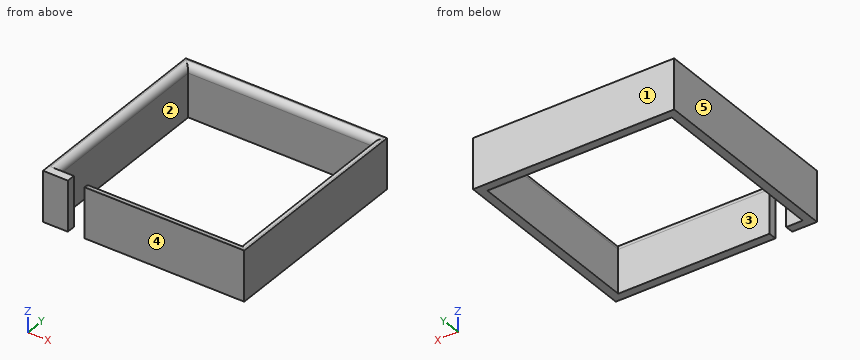
from build123d import *

# Parameters (mm, degrees)
F0_W     = 152.4
F0_H     = 152.4
F0_W_2   = 139.7
F0_H_2   = 139.7
F1_DEPTH = 38.1
F2_W     = 12.7
F2_H     = 38.1
F3_DEPTH = 37.084
F4_R     = 5.08


with BuildPart() as f1:
    # F0 (on Top) → F1 (new body)
    with BuildSketch(Plane.XY):
        with Locations((0, -7.475798)):
            Rectangle(F0_W, F0_H)
        with Locations((0, -7.475798)):
            Rectangle(F0_W_2, F0_H_2, mode=Mode.SUBTRACT)
    extrude(amount=F1_DEPTH)

    # F2 (on face) → F3 (cut)
    with BuildSketch(Plane.XZ.offset(83.675798)):
        with Locations((-51.042333, 19.05)):
            Rectangle(F2_W, F2_H)
    extrude(amount=-F3_DEPTH, mode=Mode.SUBTRACT)

    # F4
    f4_edges = [f1.edges().sort_by_distance(p)[0] for p in [
        (69.85, -7.475798, 38.1),
        (0, 62.374202, 38.1),
        (12.578834, -77.325798, 38.1),
        (-69.85, -7.475798, 38.1),
    ]]
    fillet(f4_edges, radius=F4_R)


solid = f1.part
Could you check a few things on this model? Use its own coordinates, in mm. Face numbers are marked on the shaded views. A direction names the side the tool comes from. Give positions to 0.01 mm unless a question says otherwise; leave off trailing zeros. Write each loop counter-clockwise with the first axis right and the second up, starting at its lowest first coordinate (ties: lowest second). Pieces come first, ordered by that corner, then holes. Notation, with made-up numbers: (-13, 64) -> (5, 64) arc R9 ccw to (5, 68) -> close; hole circle Ø7 at (76.5, 16). An arc over 180 degrees is marked (long way). Answer as CSV lines item,"result". Start each with the question number.
(1) If we section it at B-B, the plane y = -7: Write out the boundary of the cut face in (x, z).
(2) Please list where these lines run through material, in increasing order: line 1 (X direction, y = -10, z = 31); line 2 (Y direction, x = 30.5, z = 27.5); line 3 (Y direction, x = 69, z = 34.5).
(3) If we section it at C-C, the plane z = 16: Write out the boundary of the cut face in (x, y), and give its area (3 significant figures).
(4) Which directions (+Z, -Z, +X, -X, +Y, -Y) give clear straight access to the entire face, cutting with the end or side of a thin tool? Please do the marked faces 1 and 2.
(5) If we section it at A-A, the plane x = -32.5: Write out the boundary of the cut face in (y, z).
(6) If we mould it in two halves opening along Y, with no side actions, what happens to the marked faces 3, 4 and 5? For each: +Y half, -Y half, draft (parallel to the pull), parting line (faces both ways), or undercut.
Answer list:
1,outline,"(-76.2, 0) -> (-69.85, 0) -> (-69.85, 33.02) arc R5.08 ccw to (-74.93, 38.1) -> (-76.2, 38.1) -> close; (69.85, 0) -> (76.2, 0) -> (76.2, 38.1) -> (74.93, 38.1) arc R5.08 ccw to (69.85, 33.02) -> close"
2,line 1,"-76.2 to -69.85, 69.85 to 76.2"
2,line 2,"-83.68 to -77.33, 62.37 to 68.72"
2,line 3,"-83.68 to -77.55, 62.59 to 68.72"
3,outline,"(-76.2, -83.68) -> (-57.39, -83.68) -> (-57.39, -77.33) -> (-69.85, -77.33) -> (-69.85, 62.37) -> (69.85, 62.37) -> (69.85, -77.33) -> (-44.69, -77.33) -> (-44.69, -83.68) -> (76.2, -83.68) -> (76.2, 68.72) -> (-76.2, 68.72) -> close"
3,area,"3,630 mm^2"
4,face 1,"+Z, -Z, +X, -X, +Y"
4,face 2,"+Z, -Z"
5,outline,"(-83.68, 0) -> (-77.33, 0) -> (-77.33, 33.02) arc R5.08 ccw to (-82.41, 38.1) -> (-83.68, 38.1) -> close; (62.37, 0) -> (68.72, 0) -> (68.72, 38.1) -> (67.45, 38.1) arc R5.08 ccw to (62.37, 33.02) -> close"
6,face 3,"undercut"
6,face 4,"-Y half"
6,face 5,"draft"
